Read the model definition and answer for the solid it produces. Units are mm, in the model's axes. A direction names the side the tool comes from. Give positions to 0.01 mm unless a question says otherwise; leave off trailing zeros. Loops run counter-clockwise (first coordinate to the right, second up) from the corner with the lowest first, then second, coordinate; pieces in that order, holes last. Notation, with made-up numbers: (-0.75, 62) -> (49.25, 62) arc R21 ccw to (49.25, 90) -> close; hole circle Ø5 at (32.5, 84.25). An arc over 180 degrees is marked (long way). Write each question's results on one line, items separated by ' | '. Start each with the question number.
Item 1: Which of the six approach directions +Z, -Z, +X, -X, +Y, -Y give full straight-line access (tool end or side, diameter ignored) to faces 1 (the flat face through (12, 17.78, 12)), 2 (the cylindrical face through (-22.424, 1.574, 17.194)), 3 (the cylindrical face through (-22.424, 16.179, 17.194))?
Item 2: Section C-C on y = 8.5 is taken. Write down the section's boundary in (x, z) (1 decimal).
Item 3: Find the intervals of material crossed by line 1 (Z direction, x = 0, y = 11.75); line 2 (Z direction, x = -13, y = 6.5), in increasing order.
Item 4: Determine the mould class of faces 4 (the flat face through (12, 0, 12)), 5 (the cylindrical face through (-14.274, 9.006, -0.628)), 6 (the cylindrical face through (-6.607, 8.801, 29.755)) for opening direction X: +X half, -X half, draft (parallel to the pull), parting line (faces both ways), or undercut.
Item 5: Section B-B on z = 0 is taken. Write down the section's boundary in (x, y) (1 decimal).
Item 6: Each of these flat-tipped pins is pushed along its axis until it touches: P1, Ø2, axis at x = 6, y = 6.5, coming from the +Z side; P2, Ø1.5, axis at x = 21, z = 17, coming from the -Y side; P3, Ø6, axis at x = 20, y = 3.5, coming from the +Z side; P4, Ø10, axis at y = 9.5, z = 7.5, coming from the +X side. Where does it stop, or does it pass through?
Item 7: Section A-A on x = 0 is taken. Write down the section's boundary in (y, z) (1 decimal).
```python
from build123d import *

# Parameters (mm, degrees)
SKETCH1_R           = 28.2575
STEP_DEPTH          = 2.54
SKETCH2_R           = 30.48
BODY_DEPTH          = 12.7
SKETCH3_R           = 28.2575
BOSS_EXTRUDE3_DEPTH = 2.54
SKETCH4_R           = 14.2875
CUT_EXTRUDE1_DEPTH  = 18.78
FILLET1_R           = 0.635


with BuildPart() as part:
    # Sketch1 → Step (new body)
    with BuildSketch(Plane(origin=(0, 0, 0), x_dir=(1, 0, 0), z_dir=(0, 1, 0))):
        Circle(SKETCH1_R)
    extrude(amount=STEP_DEPTH)

    # Sketch2 → Body (add)
    with BuildSketch(Plane(origin=(0, 2.54, 0), x_dir=(1, 0, 0), z_dir=(0, 1, 0))):
        Circle(SKETCH2_R)
    extrude(amount=BODY_DEPTH)

    # Sketch3 → Boss-Extrude3 (add)
    with BuildSketch(Plane(origin=(0, 15.24, 0), x_dir=(1, 0, 0), z_dir=(0, 1, 0))):
        Circle(SKETCH3_R)
    extrude(amount=BOSS_EXTRUDE3_DEPTH)

    # Sketch4 → Cut-Extrude1 (cut, through all)
    with BuildSketch(Plane(origin=(0, 17.78, 0), x_dir=(1, 0, 0), z_dir=(0, 1, 0))):
        Circle(SKETCH4_R)
    extrude(amount=-CUT_EXTRUDE1_DEPTH, mode=Mode.SUBTRACT)

    # Fillet1
    fillet1_edges = [part.edges().sort_by_distance(p)[0] for p in [
        (-28.2575, 17.78, 0),
        (-14.2875, 0, 0),
        (-14.2875, 17.78, 0),
        (-28.2575, 0, 0),
    ]]
    fillet(fillet1_edges, radius=FILLET1_R)


solid = part.part
```
Findings:
1) face 1: +Z, -Z, +X, -X, +Y | face 2: -Y | face 3: +Y
2) outline: circle Ø61 at (0, 0); hole circle Ø28.6 at (0, 0)
3) line 1: -30.48 to -14.29, 14.29 to 30.48 | line 2: -27.57 to -5.93, 5.93 to 27.57
4) face 4: draft | face 5: undercut | face 6: parting line
5) outline: (-30.5, 2.5) -> (-28.3, 2.5) -> (-28.3, 0.6) arc R0.6 ccw to (-27.6, 0) -> (-14.9, 0) arc R0.6 ccw to (-14.3, 0.6) -> (-14.3, 17.1) arc R0.6 ccw to (-14.9, 17.8) -> (-27.6, 17.8) arc R0.6 ccw to (-28.3, 17.1) -> (-28.3, 15.2) -> (-30.5, 15.2) -> close; (14.3, 0.6) arc R0.6 ccw to (14.9, 0) -> (27.6, 0) arc R0.6 ccw to (28.3, 0.6) -> (28.3, 2.5) -> (30.5, 2.5) -> (30.5, 15.2) -> (28.3, 15.2) -> (28.3, 17.1) arc R0.6 ccw to (27.6, 17.8) -> (14.9, 17.8) arc R0.6 ccw to (14.3, 17.1) -> close
6) P1: z = 30.07 | P2: y = 0 | P3: z = 25.3 | P4: x = 30.38
7) outline: (0, -27.6) arc R0.6 ccw to (0.6, -28.3) -> (2.5, -28.3) -> (2.5, -30.5) -> (15.2, -30.5) -> (15.2, -28.3) -> (17.1, -28.3) arc R0.6 ccw to (17.8, -27.6) -> (17.8, -14.9) arc R0.6 ccw to (17.1, -14.3) -> (0.6, -14.3) arc R0.6 ccw to (0, -14.9) -> close; (0, 14.9) arc R0.6 ccw to (0.6, 14.3) -> (17.1, 14.3) arc R0.6 ccw to (17.8, 14.9) -> (17.8, 27.6) arc R0.6 ccw to (17.1, 28.3) -> (15.2, 28.3) -> (15.2, 30.5) -> (2.5, 30.5) -> (2.5, 28.3) -> (0.6, 28.3) arc R0.6 ccw to (0, 27.6) -> close
